Autodesk Inventor part; units mm, degrees
ref_plane "YZ Plane" through (0, 0, 0) normal (1, 0, 0) x (0, 1, 0)
ref_plane "XZ Plane" through (0, 0, 0) normal (0, 1, 0) x (-1, 0, 0)
ref_plane "XY Plane" through (0, 0, 0) normal (0, 0, 1) x (1, 0, 0)
sketch "Sketch1" plane through (0, 0, 0) normal (0, 0, 1) x (1, 0, 0)
  line L0 (0, 0) -> (0, 1479.6195)
  line L1 (0, 1479.6195) -> (-166.4399, 1479.6195)
  line L2 (-166.4399, 1479.6195) -> (-200, 0)
  line L3 (-200, 0) -> (0, 0)
  line L4 (0, 430) -> (-5, 430)
  line L5 (-5, 430) -> (-5, 368)
  line L6 (-5, 368) -> (0, 368)
  line L7 (0, 368) -> (0, 430)
  line L8 (-5, 430) -> (-70, 430)
  line L9 (-70, 430) -> (-70, 425)
  line L10 (-70, 425) -> (-5, 425)
  line L11 (-5, 425) -> (-5, 430)
  line L12 (-70, 430) -> (-190.2469, 430) construction
  line L13 (0, 4408.8661) -> (0, 1479.6195)
  line L14 (-166.4399, 1479.6195) -> (-132.8798, 2959.2389)
  line L15 (0, 4408.8661) -> (-100, 4408.8661)
  line L16 (-132.8798, 2959.2389) -> (0, 2959.2389)
  line L17 (-132.8798, 2959.2389) -> (-100, 4408.8661)
  line L18 (-5, 868) -> (0, 868)
  line L19 (-70, 925) -> (-5, 925)
  line L20 (-5, 930) -> (-70, 930)
  line L21 (-70, 930) -> (-70, 925)
  line L22 (-5, 925) -> (-5, 930)
  line L23 (-5, 930) -> (-5, 868)
  line L24 (0, 868) -> (0, 930)
  line L25 (0, 930) -> (-5, 930)
  line L26 (-5, 1368) -> (0, 1368)
  line L27 (-70, 1425) -> (-5, 1425)
  line L28 (-5, 1430) -> (-70, 1430)
  line L29 (-70, 1430) -> (-70, 1425)
  line L30 (-5, 1425) -> (-5, 1430)
  line L31 (-5, 1430) -> (-5, 1368)
  line L32 (0, 1368) -> (0, 1430)
  line L33 (0, 1430) -> (-5, 1430)
  line L34 (-5, 1868) -> (0, 1868)
  line L35 (-70, 1925) -> (-5, 1925)
  line L36 (-5, 1930) -> (-70, 1930)
  line L37 (-70, 1930) -> (-70, 1925)
  line L38 (-5, 1925) -> (-5, 1930)
  line L39 (-5, 1930) -> (-5, 1868)
  line L40 (0, 1868) -> (0, 1930)
  line L41 (0, 1930) -> (-5, 1930)
  line L42 (-5, 2368) -> (0, 2368)
  line L43 (-70, 2425) -> (-5, 2425)
  line L44 (-5, 2430) -> (-70, 2430)
  line L45 (-70, 2430) -> (-70, 2425)
  line L46 (-5, 2425) -> (-5, 2430)
  line L47 (-5, 2430) -> (-5, 2368)
  line L48 (0, 2368) -> (0, 2430)
  line L49 (0, 2430) -> (-5, 2430)
  line L50 (-5, 2868) -> (0, 2868)
  line L51 (-70, 2925) -> (-5, 2925)
  line L52 (-5, 2930) -> (-70, 2930)
  line L53 (-70, 2930) -> (-70, 2925)
  line L54 (-5, 2925) -> (-5, 2930)
  line L55 (-5, 2930) -> (-5, 2868)
  line L56 (0, 2868) -> (0, 2930)
  line L57 (0, 2930) -> (-5, 2930)
  line L58 (-100, 4408.8661) -> (-99.3197, 4438.8584) construction
  line L59 (0, 1629.6195) -> (-163.0377, 1629.6195)
  line L60 (-131.0653, 3039.2389) -> (0, 3039.2389)
  line L61 (-5, 3368) -> (0, 3368)
  line L62 (-70, 3425) -> (-5, 3425)
  line L63 (-5, 3430) -> (-70, 3430)
  line L64 (-70, 3430) -> (-70, 3425)
  line L65 (-5, 3425) -> (-5, 3430)
  line L66 (-5, 3430) -> (-5, 3368)
  line L67 (0, 3368) -> (0, 3430)
  line L68 (0, 3430) -> (-5, 3430)
  line L69 (-5, 3868) -> (0, 3868)
  line L70 (-70, 3925) -> (-5, 3925)
  line L71 (-5, 3930) -> (-70, 3930)
  line L72 (-70, 3930) -> (-70, 3925)
  line L73 (-5, 3925) -> (-5, 3930)
  line L74 (-5, 3930) -> (-5, 3868)
  line L75 (0, 3868) -> (0, 3930)
  line L76 (0, 3930) -> (-5, 3930)
  arc A0 (-140, 0) -> (-198.6395, 59.9846) centre (-200, 0) ccw
  arc A1 (-167.1202, 1449.6272) -> (-165.7596, 1509.6117) centre (-166.4399, 1479.6195) ccw
  arc A2 (-133.5601, 2929.2466) -> (-132.1995, 2989.2312) centre (-132.8798, 2959.2389) ccw
  line L77 (0, 930) -> (-70, 930)
  line L78 (-70, 930) -> (-178.9061, 930) construction
  line L79 (-70, 1430) -> (-167.5654, 1430) construction
  line L80 (-70, 1930) -> (-156.2246, 1930) construction
  line L81 (-70, 2430) -> (-144.8838, 2430) construction
  line L82 (-70, 2930) -> (-133.543, 2930) construction
  line L83 (-70, 3430) -> (-122.2022, 3430) construction
  line L84 (-70, 3930) -> (-110.8614, 3930) construction
  point P0 (0, 430)
  point P1 (-136.4399, 1479.6195)
  point P2 (0, 2368)
  point P3 (0, 2868)
  point P4 (0, 1868)
  point P5 (-102.8798, 2959.2389)
  point P6 (0, 3368)
  point P7 (0, 3868)
  dimension "d25" = 430
  dimension "d32" = 1480
  dimension "d33" = 1480
  dimension "d34" = 1450
  dimension "d35" = 100
  dimension "d38" = 500
  dimension "d44" = 30
  dimension "d45" = 150
  dimension "d46" = 80
  dimension "d47" = 200
  dimension "d48" = 5
  dimension "d50" = 62
  dimension "d51" = 60
  dimension "d52" = 30
  dimension "d53" = 478.8661
  dimension "d54" = 30
  dimension "d56" = 190.2469
  dimension "d57" = 178.9061
  dimension "d58" = 167.5654
  dimension "d59" = 156.2246
  dimension "d60" = 144.8838
  dimension "d61" = 133.543
  dimension "d62" = 122.2022
  dimension "d63" = 110.8614
  dimension "d64" = 70
extrude "Plate1" add sketch "Sketch1" along normal blind 4 contours A2 L17 L60 L13 L16 | L17 L15 L13 L76 L71 L72 L70 L74 L69 L68 L63 L64 L62 L66 L61 L60
sketch "Sketch2" plane through (4, 4408.8661, 0) normal (-1, 0, 0) x (0, -1, 0)
  line L0 (478.8661, 0) -> (0, 0)
  line L1 (0, 0) -> (0, 50)
  line L2 (0, 50) -> (478.8661, 50)
  line L3 (478.8661, 50) -> (478.8661, 0)
edge flange "Flange1" height 50 angle 90 thickness 4 bend radius 4 thickness toward (-1, 0, 0) relief tear relief width 4 relief depth 2 corner gap 4 corner form 0 edges at (0, 4169.433, 4) (0, 3649, 4) (0, 3163.6195, 4) wall of the first edge with corners at (4, 3930, 0) (4, 4408.8661, 0) (4, 4408.8661, 50) (4, 3930, 50)
bend "Bend1"
corner "Corner1"
chamfer "Corner Chamfer1" distance 6 angle 45 2 edges at (-5, 3425, 2) (-5, 3925, 2)
equation "\"d5\" = Thickness"
equation "\"d7\" = BendReliefWidth"
equation "\"d8\" = BendReliefDepth"
equation "\"d9\" = MinimumRemnant"
equation "\"d10\" = TransitionRadius"
equation "\"d13\" = BendRadius"
equation "\"d14\" = CornerReliefSize"
equation "\"d15\" = GapSize"
equation "\"d16\" = JacobiRadiusSize"
equation "\"BendRadius\" = Thickness"
equation "\"BendReliefWidth\" = Thickness"
equation "\"BendReliefDepth\" = 0.5 * Thickness"
equation "\"CornerReliefSize\" = 4 * Thickness"
equation "\"MinimumRemnant\" = 2 * Thickness"
equation "\"TransitionRadius\" = BendRadius"
equation "\"JacobiRadiusSize\" = BendRadius"
equation "\"GapSize\" = Thickness"
properties part number "03.1 GBK main3  rib" material "Steel"
Read the model definition and answer for the solid it produces. Units are mm, in the model's axes. A direction names the side the tool comes from. Give positions to 0.01 mm unless a question says otherwise; leave off trailing zeros. Write each loop counter-clockwise with the first axis right and the second up, starting at its lowest first coordinate (ties: lowest second). Pieces come first, ordered by that corner, then holes. Notation, with made-up numbers: (-5.5, 6.25) -> (27.5, 6.25) arc R12 cw to (27.5, 27.25) -> close; hole circle Ø11 at (-1, 31). An arc over 180 degrees is marked (long way). Answer as a JSON object with one key per item and string values. Group by question number.
1) A tool of negligible diameter and unlimited length cuts with its end or side. For faces 4 (the flat face through (0, 4173, 29)), 5 (the flat face through (-34, 2959.239, 3)), 6 (the flat face through (-16, 3430, 3)), from which of +Z, -Z, +X, -X, +Y, -Y can it reach the whole face along a straight path? Write none if from no direction.
2) Consider L1, parallel to Z at x = -6.5, y = 4190; L2, parallel to X at y = 3859.5, z = 7. Determine where each line is inside the solid, lowest interval first. Write a range as from..to.
3) Find section A-A (x = -53). Write down the section's boundary in (y, z), and give its area (3 significant figures).
4) Find section C-C (y = 3092). Write down the section's boundary in (x, z).
5) Each of these flat-tipped pins is pushed along its axis until it touches: P1, Ø2, axis at y = 3928, z = 2, coming from the +X side; P2, Ø3, axis at x = -81, y = 3235, coming from the +Z side; P3, Ø2.5, axis at x = -2.5, z = 35.5, coming from the +Y side; P4, Ø6, axis at y = 4259, z = 10.5, coming from the -X side. Where does it stop, or does it pass through?
6) The mould has two halves that part along Y. Classify faces 1 (the flat face through (-16, 3930, 3)), 2 (the flat face through (4, 3166, 29)), 3 (the flat face through (-32, 4408.866, 3)): +Y half, -Y half, draft (parallel to the pull), parting line (faces both ways), or undercut.
7) Find section B-B (z = 27). Write down the section's boundary in (x, y).
8) Find section D-D (y = 3713). Write down the section's boundary in (x, z).
Values follow:
{
 "1": {"face 4": "+Z, -X, +Y, -Y", "face 5": "+Z, -Z, +X, -X, -Y", "face 6": "+Z, -Z, +X"},
 "2": {"L1": "z = 0..4", "L2": "x = -0.13..3.94"},
 "3": {"outline": "(2959.24, 0) -> (3425, 0) -> (3425, 4) -> (2959.24, 4) -> close; (3430, 0) -> (3925, 0) -> (3925, 4) -> (3430, 4) -> close; (3930, 0) -> (4408.87, 0) -> (4408.87, 4) -> (3930, 4) -> close", "area": "5,760 mm2"},
 "4": {"outline": "(-129.87, 0) -> (-4, 0) arc R8 ccw to (4, 8) -> (4, 50) -> (0, 50) -> (0, 8) arc R4 cw to (-4, 4) -> (-129.87, 4) -> close"},
 "5": {"P1": "stops at x = -70", "P2": "stops at z = 4", "P3": "passes through", "P4": "stops at x = -0.03"},
 "6": {"face 1": "undercut", "face 2": "draft", "face 3": "+Y half"},
 "7": {"outline": "(0, 2959.24) -> (4, 2959.24) -> (4, 3368) -> (0, 3368) -> close; (0, 3430) -> (4, 3430) -> (4, 3868) -> (0, 3868) -> close; (0, 3930) -> (4, 3930) -> (4, 4408.87) -> (0, 4408.87) -> close"},
 "8": {"outline": "(-115.78, 0) -> (-4, 0) arc R8 ccw to (4, 8) -> (4, 50) -> (0, 50) -> (0, 8) arc R4 cw to (-4, 4) -> (-115.78, 4) -> close"}
}
